Could you check a few things on this model? Use its own coordinates, in mm. Face numbers are marked on the shaded views. A direction names the side the tool comes from. Give positions to 0.01 mm unless a question says otherwise; leave off trailing zeros. Order: outer loops, then holes, each group sorted by start corner. A loop starts at its lowest first (then second) coordinate and runs counter-clockwise, first axis right, second up. Notation, with made-up numbers: (24, -0.5) - (70, -0.5) arc R24 cw to (70, 11.5) - close; hole circle Ø4 at (59.5, 11.25). An arc over 180 degrees is marked (long way). One line per question, with ' | ' between items. Start each with the question number.
1. Imagine slicing it at C-C (y = 4). Please give me the cut outline in (x, z).
2. Imagine slicing it at D-D (z = -32). Please give me the cut outline in (x, y).
3. Which directions (+Z, -Z, +X, -X, +Y, -Y) give clear straight access to the entire face, cutting with the end or side of a thin tool? Please do the marked faces 1, 2 and 3.
4. For P1, Ø1, axis at y = 4.5, z = 53.5, coming from the +X side; P2, Ø8, axis at x = 0, z = -57, coming from the +Y side; P3, Ø1, axis at x = 29, y = 13, coming from the +Z side, each with a flat end and sliding along its axis, tell me the tip position at first contact or that it passes through.
5. Imagine slicing it at A-A (z = -57). Please give me the cut outline in (x, y), and give its area (3 significant figures).
6. I need wall thicknesses on probe 1 along X at (y, z) = (-2.7, -57); probe 2 along X at (y, z) = (9.25, -49); probe 3 along Z at (x, y) = (-17.5, 10.5). Which ranges of each line are inside material? Lowest first, please. Write a range as from..to.
7. Imagine slicing it at B-B (x = 0). Please give me the cut outline in (y, z).
8. If we mould it in two halves opening along Z, with no side actions, what happens to the marked faces 4, 5, 6 and 7? For each: released by +Z, released by -Z, zero draft, split by the parting line, or undercut.
```python
from build123d import *

# Parameters (mm, degrees)
SKETCH1_W               = 80
SKETCH1_H               = 94
SKETCH1_W_2             = 72
SKETCH1_H_2             = 86
BOSS_EXTRUDE3_DEPTH     = 20
SKETCH10_W              = 80
SKETCH10_H              = 134
BOSS_EXTRUDE4_DEPTH     = 4
CUT_EXTRUDE1_REACH      = 108.25
SKETCH11_W              = 10
SKETCH11_H              = 20
FILLET2_R               = 2
TAP_DRILL_FOR_M8_TAP2_D = 6.8
RIB10_REACH             = 94.79
SKETCH26_WALL_W         = 215.864442602
SKETCH26_WALL_H         = 4
MIRROR4_COPY_1_REACH    = 94.79
MIRROR4_COPY_1_SKETCH_W = 215.864442602
MIRROR4_COPY_1_SKETCH_H = 4
CHAMFER1_SIZE           = 5


with BuildPart() as part:
    # Sketch1 → Boss-Extrude3 (new body)
    with BuildSketch(Plane(origin=(0, 0, 0), x_dir=(1, 0, 0), z_dir=(0, 1, 0))):
        Rectangle(SKETCH1_W, SKETCH1_H)
        Rectangle(SKETCH1_W_2, SKETCH1_H_2, mode=Mode.SUBTRACT)
    extrude(amount=BOSS_EXTRUDE3_DEPTH)

    # Sketch10 → Boss-Extrude4 (add)
    with BuildSketch(Plane.XZ):
        Rectangle(SKETCH10_W, SKETCH10_H)
    extrude(amount=BOSS_EXTRUDE4_DEPTH)

    # Sketch11 → Cut-Extrude1 (cut, up to next)
    with BuildSketch(Plane.ZY.offset(40), mode=Mode.PRIVATE) as cut_extrude1_sk1:
        with Locations((0, 10)):
            Rectangle(SKETCH11_W, SKETCH11_H)
    cut_extrude1_tool1 = extrude(cut_extrude1_sk1.sketch, amount=-CUT_EXTRUDE1_REACH, mode=Mode.PRIVATE) & part.part
    add(cut_extrude1_tool1.solids().sort_by_distance((-40, 10, 0))[0], mode=Mode.SUBTRACT)

    # Fillet2
    fillet2_edges = [part.edges().sort_by_distance(p)[0] for p in [
        (-38, 20, 5),
        (-38, 20, -5),
    ]]
    fillet(fillet2_edges, radius=FILLET2_R)

    # Tap Drill for M8 Tap2 (through all)
    with Locations(Plane(origin=(0, 0, 57), x_dir=(0, 0, 1), z_dir=(0, 1, 0))):
        with Locations((0, 0), (-114, 0)):
            Hole(TAP_DRILL_FOR_M8_TAP2_D / 2)

    # Sketch26 wall → Rib10 (add, up to next)
    with BuildSketch(Plane(origin=(-21, 10, -57), x_dir=(0, 0.707106781187, 0.707106781187), z_dir=(0, 0.707106781187, -0.707106781187)), mode=Mode.PRIVATE) as rib10_sk1:
        Rectangle(SKETCH26_WALL_W, SKETCH26_WALL_H)
    rib10_tool1 = extrude(rib10_sk1.sketch, amount=-RIB10_REACH, mode=Mode.PRIVATE) - part.part
    rib10 = rib10_tool1.solids().sort_by_distance((-21, 10, -57))[0]
    add(rib10)

    # Mirror3: Rib10 across plane
    add(rib10.mirror(Plane(origin=(0, 0, 0), x_dir=(0, 0, 1), z_dir=(1, 0, 0))))

    # Mirror4: Rib10 across plane
    add(rib10.mirror(Plane.XY))

    # Mirror4 copy 1 sketch → Mirror4 copy 1 (add, up to next)
    with BuildSketch(Plane(origin=(21, 10, 57), x_dir=(0, 0.707106781187, -0.707106781187), z_dir=(0, 0.707106781187, 0.707106781187)), mode=Mode.PRIVATE) as mirror4_copy_1_sk1:
        Rectangle(MIRROR4_COPY_1_SKETCH_W, MIRROR4_COPY_1_SKETCH_H)
    mirror4_copy_1_tool1 = extrude(mirror4_copy_1_sk1.sketch, amount=-MIRROR4_COPY_1_REACH, mode=Mode.PRIVATE) - part.part
    add(mirror4_copy_1_tool1.solids().sort_by_distance((21, 10, 57))[0])

    # Chamfer1
    chamfer1_edges = [part.edges().sort_by_distance(p)[0] for p in [
        (40, -2, -67),
        (40, -2, 67),
        (-40, -2, 67),
        (-40, -2, -67),
    ]]
    chamfer(chamfer1_edges, length=CHAMFER1_SIZE)


solid = part.part
```
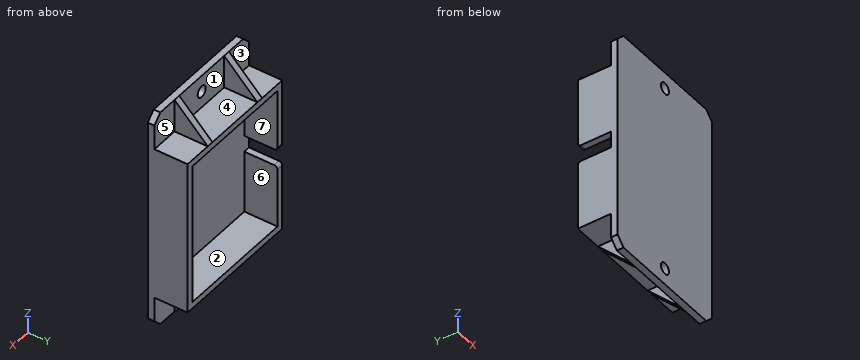
Results found:
1) outline: (-40, -47) - (-23, -47) - (-23, -63) - (-19, -63) - (-19, -47) - (19, -47) - (19, -63) - (23, -63) - (23, -47) - (40, -47) - (40, 47) - (23, 47) - (23, 63) - (19, 63) - (19, 47) - (-19, 47) - (-19, 63) - (-23, 63) - (-23, 47) - (-40, 47) - (-40, 5) - (-36, 5) - (-36, 43) - (36, 43) - (36, -43) - (-36, -43) - (-36, -5) - (-40, -5) - close
2) outline: (-40, -4) - (40, -4) - (40, 20) - (36, 20) - (36, 0) - (-36, 0) - (-36, 20) - (-40, 20) - close
3) face 1: +Z, +Y | face 2: +Y | face 3: +Z, -X, +Y
4) P1: stops at x = 23 | P2: stops at y = 0 | P3: stops at z = 47
5) outline: (-40, -4) - (-3.4, -4) - (-3.4, 0) - (-19, 0) - (-19, 10) - (-23, 10) - (-23, 0) - (-40, 0) - close; (3.4, -4) - (40, -4) - (40, 0) - (23, 0) - (23, 10) - (19, 10) - (19, 0) - (3.4, 0) - close | area: 373 mm2
6) probe 1: x = -40..-3.4, 3.4..40 | probe 2: x = -23..-19, 19..23 | probe 3: z = -47..-43, 43..47
7) outline: (-4, -67) - (0, -67) - (0, -60.4) - (-4, -60.4) - close; (-4, -53.6) - (0, -53.6) - (0, -47) - (20, -47) - (20, -43) - (0, -43) - (0, 43) - (20, 43) - (20, 47) - (0, 47) - (0, 53.6) - (-4, 53.6) - close; (-4, 60.4) - (0, 60.4) - (0, 67) - (-4, 67) - close
8) face 4: released by +Z | face 5: zero draft | face 6: undercut | face 7: undercut
